```python
from build123d import *

# Parameters (mm, degrees)
SKETCH1_W                = 50
SKETCH1_H                = 35
BOSS_EXTRUDE1_DEPTH      = 40
CUT_EXTRUDE3_DEPTH       = 15
CUT_EXTRUDE6_DEPTH       = 51.311529494
CUT_EXTRUDE6_DEPTH_BACK  = 51.311529494
CUT_EXTRUDE8_DEPTH       = 51.292408862
CUT_EXTRUDE8_DEPTH_BACK  = 51.292408862
SKETCH6_W                = 40
SKETCH6_H                = 12.54309885
CUT_EXTRUDE9_DEPTH       = 25
SKETCH7_R                = 1.25
CUT_EXTRUDE10_DEPTH      = 51.292408862
CUT_EXTRUDE10_DEPTH_BACK = 51.292408862


with BuildPart() as part:
    # Sketch1 → Boss-Extrude1 (new body)
    with BuildSketch(Plane.XY):
        Rectangle(SKETCH1_W, SKETCH1_H)
    extrude(amount=BOSS_EXTRUDE1_DEPTH)

    # Sketch3 → Cut-Extrude3 (cut)
    with BuildSketch(Plane.XY):
        with BuildLine():
            ThreePointArc((18.080023646, 4.616675297), (22.774898037, 4.159319762), (25, 0))
            Line((25, 0), (25, 17.5))
            Line((25, 17.5), (20.265083079, 17.5))
            ThreePointArc((20.265083079, 17.5), (22.164558634, 14.89755515), (22.836723839, 11.746536186))
            ThreePointArc((22.836723839, 11.746536186), (21.538401387, 7.461063254), (18.080023646, 4.616675297))
        make_face()
        with BuildLine():
            ThreePointArc((9.964651512, 17.5), (7.890776302, 14.474095131), (7.447285057, 10.832615462))
            ThreePointArc((7.447285057, 10.832615462), (11.217729841, 5.080248753), (18.080023646, 4.616675297))
            ThreePointArc((18.080023646, 4.616675297), (21.538401387, 7.461063254), (22.836723839, 11.746536186))
            ThreePointArc((22.836723839, 11.746536186), (22.164558634, 14.89755515), (20.265083079, 17.5))
            Line((20.265083079, 17.5), (9.964651512, 17.5))
        make_face()
        with BuildLine():
            ThreePointArc((20.265083079, 17.5), (15.114867296, 19.46839273), (9.964651512, 17.5))
            Line((9.964651512, 17.5), (20.265083079, 17.5))
        make_face()
        with BuildLine():
            ThreePointArc((-7.393010752, 11.746536186), (-7.406591271, 11.28877073), (-7.447285061, 10.832615429))
            ThreePointArc((-7.447285061, 10.832615429), (-1.7e-08, 17.444952642), (7.447285057, 10.832615462))
            ThreePointArc((7.447285057, 10.832615462), (7.890776302, 14.474095131), (9.964651512, 17.5))
            Line((9.964651512, 17.5), (-9.964651512, 17.5))
            ThreePointArc((-9.964651512, 17.5), (-8.065175957, 14.89755515), (-7.393010752, 11.746536186))
        make_face()
        with BuildLine():
            ThreePointArc((-20.265083079, 17.5), (-22.728002657, 10.455320307), (-18.080023619, 4.616675286))
            ThreePointArc((-18.080023619, 4.616675286), (-11.217729842, 5.080248753), (-7.447285061, 10.832615429))
            ThreePointArc((-7.447285061, 10.832615429), (-7.406591271, 11.28877073), (-7.393010752, 11.746536186))
            ThreePointArc((-7.393010752, 11.746536186), (-8.065175957, 14.89755515), (-9.964651512, 17.5))
            Line((-9.964651512, 17.5), (-20.265083079, 17.5))
        make_face()
        with BuildLine():
            ThreePointArc((-9.964651512, 17.5), (-15.114867296, 19.46839273), (-20.265083079, 17.5))
            Line((-20.265083079, 17.5), (-9.964651512, 17.5))
        make_face()
        with BuildLine():
            Line((-25, 17.5), (-25, 2.5e-08))
            ThreePointArc((-25, 2.5e-08), (-22.774898014, 4.159319778), (-18.080023619, 4.616675286))
            ThreePointArc((-18.080023619, 4.616675286), (-22.728002657, 10.455320307), (-20.265083079, 17.5))
            Line((-20.265083079, 17.5), (-25, 17.5))
        make_face()
    extrude(amount=CUT_EXTRUDE3_DEPTH, mode=Mode.SUBTRACT)

    # Sketch4 → Cut-Extrude6 (cut, two sides)
    with BuildSketch(Plane(origin=(0, 0, 0), x_dir=(0, 0, -1), z_dir=(1, 0, 0))) as cut_extrude6_sk:
        with BuildLine():
            add(Edge.make_bspline(
                [(-9.222271241, 17.444952642), (-10.649134008, 17.379362556), (-16.532124994, 16.800094175), (-24.99058992, 11.744877304), (-33.962260097, 3.205152878), (-39.211523546, -3.38022438), (-40, -7.980712731)],
                knots=[0.128951398, 0.128951398, 0.128951398, 0.128951398, 0.217673321, 0.497466286, 0.713557135, 1, 1, 1, 1], degree=3))
            Line((-9.222271241, 17.444952642), (-40, 17.444952642))
            Line((-40, 17.444952642), (-40, -7.980712731))
        make_face()
        with BuildLine():
            Line((0, 0), (-3.44001081, -7.539638425))
            ThreePointArc((-3.44001081, -7.539638425), (-10.74719823, -12.539419504), (-17.727021343, -7.091955125))
            add(Edge.make_bspline(
                [(-17.727021343, -7.091955125), (-18.502936425, -5.824551955), (-21.808604968, -4.479724911), (-27.869116221, -5.844724863), (-33.812288914, -9.39721757), (-39.72251086, -14.860797268), (-40, -9.623944384)],
                knots=[0.042605041, 0.042605041, 0.042605041, 0.042605041, 0.193253168, 0.379939411, 0.648785626, 0.970666237, 0.970666237, 0.970666237, 0.970666237], degree=3))
            Line((-40, -9.623944384), (-40, -17.5))
            Line((-40, -17.5), (0, -17.5))
            Line((0, -17.5), (0, 0))
        make_face()
    extrude(amount=CUT_EXTRUDE6_DEPTH, mode=Mode.SUBTRACT)
    extrude(cut_extrude6_sk.sketch, amount=-CUT_EXTRUDE6_DEPTH_BACK, mode=Mode.SUBTRACT)


with BuildPart() as cut_extrude6_kept_piece:
    # of the separate pieces the step leaves, the one the design keeps (cut_extrude6_pieces_kept)
    add(part.part.solids().sort_by_distance((-7.447285061, 10.832615429, 15))[0])

    # Sketch5 → Cut-Extrude8 (cut, two sides)
    with BuildSketch(Plane(origin=(0, 0, 0), x_dir=(1, 0, 0), z_dir=(0, 1, 0))) as cut_extrude8_sk:
        with BuildLine():
            add(Edge.make_bspline(
                [(-25, -12.617742903), (-21.837163113, -31.626777816), (0, -40.051194025)],
                knots=[0, 0, 0, 1, 1, 1], degree=2))
            Line((0, -40.051194025), (-25, -40))
            Line((-25, -40), (-25, -12.617742903))
        make_face()
        with BuildLine():
            Line((25, -40), (25, -12.617742903))
            add(Edge.make_bspline(
                [(25, -12.617742903), (21.837163113, -31.626777816), (0, -40.051194025)],
                knots=[0, 0, 0, 1, 1, 1], degree=2))
            Line((0, -40.051194025), (25, -40))
        make_face()
    extrude(amount=CUT_EXTRUDE8_DEPTH, mode=Mode.SUBTRACT)
    extrude(cut_extrude8_sk.sketch, amount=-CUT_EXTRUDE8_DEPTH_BACK, mode=Mode.SUBTRACT)

    # Sketch6 → Cut-Extrude9 (cut)
    with BuildSketch(Plane.XY):
        with Locations((0, -6.271549425)):
            Rectangle(SKETCH6_W, SKETCH6_H)
    extrude(amount=CUT_EXTRUDE9_DEPTH, mode=Mode.SUBTRACT)

    # Sketch7 → Cut-Extrude10 (cut, two sides)
    with BuildSketch(Plane(origin=(0, 0, 0), x_dir=(0, 0, -1), z_dir=(1, 0, 0))) as cut_extrude10_sk:
        with Locations((-10.065545273, -8.297943519)):
            Circle(SKETCH7_R)
    extrude(amount=CUT_EXTRUDE10_DEPTH, mode=Mode.SUBTRACT)
    extrude(cut_extrude10_sk.sketch, amount=-CUT_EXTRUDE10_DEPTH_BACK, mode=Mode.SUBTRACT)


solid = cut_extrude6_kept_piece.part
```
Source: CAD feature listing. Evaluate the final solid. Frame: model axes, mm. A direction names the side the tool comes from. Give positions to 0.01 mm unless a question says otherwise; leave off trailing zeros. Use a Markdown table: item, result.
Q1. Material intervals for line 1 (X direction, y = -8.25, z = 7.5); line 2 (X direction, y = -5, z = 18.5); line 3 (Z direction, x = -19, y = 8.25), sorted ascending. Write a range as [from, to].
A:
| item | result |
|---|---|
| line 1 | [-25, -20], [20, 25] |
| line 2 | [-23.48, -20], [20, 23.48] |
| line 3 | [15, 26.78] |
Q2. Access query for faces 5 (the face through (0, 0, 12)), 6 (the face through (22.535, -3.717, 1.696)), 7 (the face through (-0.152, 17.443, 7.395)). Directions: +Z, -Z, +X, -X, +Y, -Y. A direction counts if a zero-diameter tool reaches every point of the face in a straight line with its end or side. Return the directions, or none.
A:
| item | result |
|---|---|
| face 5 | -Z, -Y |
| face 6 | -Z, +X, -X, -Y |
| face 7 | -Z, +Y |
Q3. Section A-A (z = 10). State how many separate pieces and enclosed holes the cut face has, and give its area (3 significant figures).
A:
| item | result |
|---|---|
| separate pieces | 3 |
| enclosed holes | 0 |
| area | 506 mm^2 |
Q4. First-contact query: P1, Ø2, axis at y = -6, z = 32.5, coming from the +X side; P2, Ø12, axis at x = 5, z = 25, coming from the +Y side; P3, Ø6, axis at x = -1, y = -4, coming from the -Z side; P4, Ø2, axis at y = -8.3, z = 10.07, coming from the -X side. Flat tips, straight axial feed; report the tip coordinate or a pass-through.
A:
| item | result |
|---|---|
| P1 | x = 14.62 |
| P2 | y = 14.97 |
| P3 | z = 25 |
| P4 | through |
Q5. Pull-direction query (Z, two-part tool) for faces 1 (the face through (-22.465, -9.059, 11.058)), 2 (the face through (22.465, -9.059, 11.058)), 3 (the face through (11.13, 5.13, 7.4)), 4 (the face through (0, -3, 25)); classes: +Z half, -Z half, draft (parallel to the pull), parting line (faces both ways), or undercut.
A:
| item | result |
|---|---|
| face 1 | undercut |
| face 2 | undercut |
| face 3 | draft |
| face 4 | -Z half |
